Check sheet for the drawn part. Datum: minimum x, y, z corner. Units: mm. A direction names the side the tool comes from. Give positions to 0.01 mm unless a question says otherwise; leave off trailing zeros. Loops run counter-clockwise (first coordinate to the right, second up) from the corner with the lowest first, then second, coordinate; pieces in that order, holes last. Notation, with made-up numbers: (-39.5, 59.5) -> (1.5, 59.5) arc R31 ccw to (1.5, 83.5) -> close; hole circle Ø3 at (77.25, -20.5). An arc over 180 degrees is marked (long way). One line per question, with ' | ' between items.
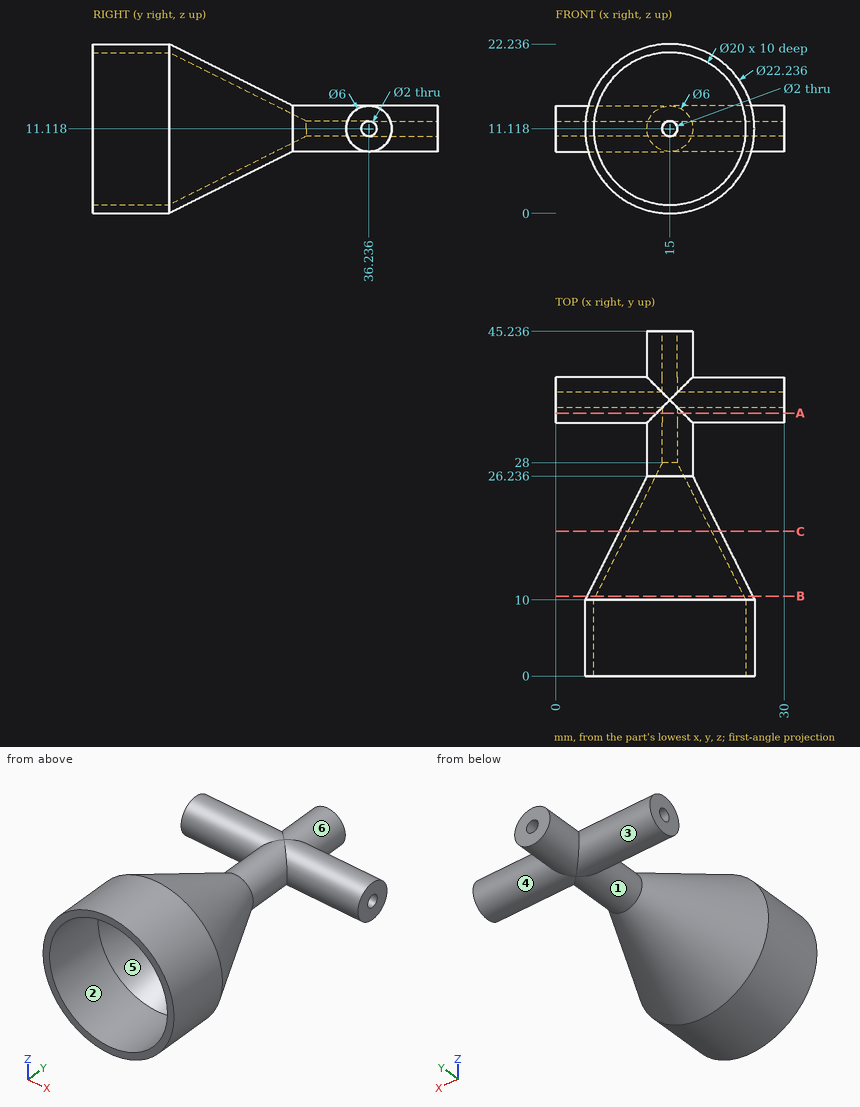
Item 1: Sectioned sample at C-C (y = 19). Record the cut outline in (x, z).
Result:
outline: circle Ø13.24 at (15, 11.12); hole circle Ø11 at (15, 11.12)
Item 2: Scan lines: probe 1 along Z at (x, y) = (15, 3.5); probe 2 along Z at (x, y) = (15, 30); probe 3 along Y at (x, z) = (13, 8.75) (1 decimal). Record each from-to range of solid material in increasing order.
Result:
probe 1: 0 to 1.12, 21.12 to 22.24 | probe 2: 8.12 to 10.12, 12.12 to 14.12 | probe 3: 23.8 to 26, 34.4 to 38.1
Item 3: Sectioned sample at A-A (y = 34.5). Record the cut outline in (x, z), plus the area to 3 significant figures.
Result:
outline: (0, 8.67) -> (13.26, 8.67) arc R3 ccw to (16.74, 8.67) -> (30, 8.67) -> (30, 13.56) -> (16.74, 13.56) arc R3 ccw to (13.26, 13.56) -> (0, 13.56) -> close; hole circle Ø2 at (15, 11.12) | area: 146 mm2
Item 4: Release check for a two-part mould opening along Y. For the marked faces 4, 5 and 6 record: pulls with the +Y half, pulls with the -Y half, needs draft (parallel to the pull), parting line crosses it, or undercut.
Result:
face 4: undercut | face 5: pulls with the -Y half | face 6: needs draft
Item 5: Sectioned sample at B-B (y = 10.5). Record the cut outline in (x, z).
Result:
outline: circle Ø21.74 at (15, 11.12); hole circle Ø19.5 at (15, 11.12)
Item 6: Set-up check for the marked faces 1, 2 and 3: record each of +Z, -Z, +X, -X, +Y, -Y from which the full face is reachable in a straight line by a thin tool's end or side.
Result:
face 1: none | face 2: -Y | face 3: -X
Item 7: Depth check by flat-ended pin: pin 1 Ø5 at (x, y) = (11, 7.5) entering from +Z; pin 2 Ø1.5 at (x, z) = (18.5, 15.5) entering from +Y; pin 3 Ø1.8 at (x, z) = (15, 11.118) entering from -Y; pin 4 Ø1 at (x, z) = (8.5, 3) entering from +Y. Enter the tip coordinate at first touch or a pass-through.
Result:
pin 1: z = 22.13 | pin 2: y = 22.52 | pin 3: through | pin 4: y = 12.44
